For this review, use the dimensioned drawing (mm, ordinates from the lowest corner) and the shaded views. A direction names the side the tool comes from. Coordinates: 2 decimals unless noted, no trailing zeros. Loops run counter-clockwise (first coordinate to the right, second up) from the corner with the lowest first, then second, coordinate; pieces in that order, holes last. Notation, with made-up numbers: M 64,43 L 83,43 A31 ccw 83,71 Z; hole C 43.25,32.5 d5. An arc over 180 degrees is marked long. One line per item, written item: value.
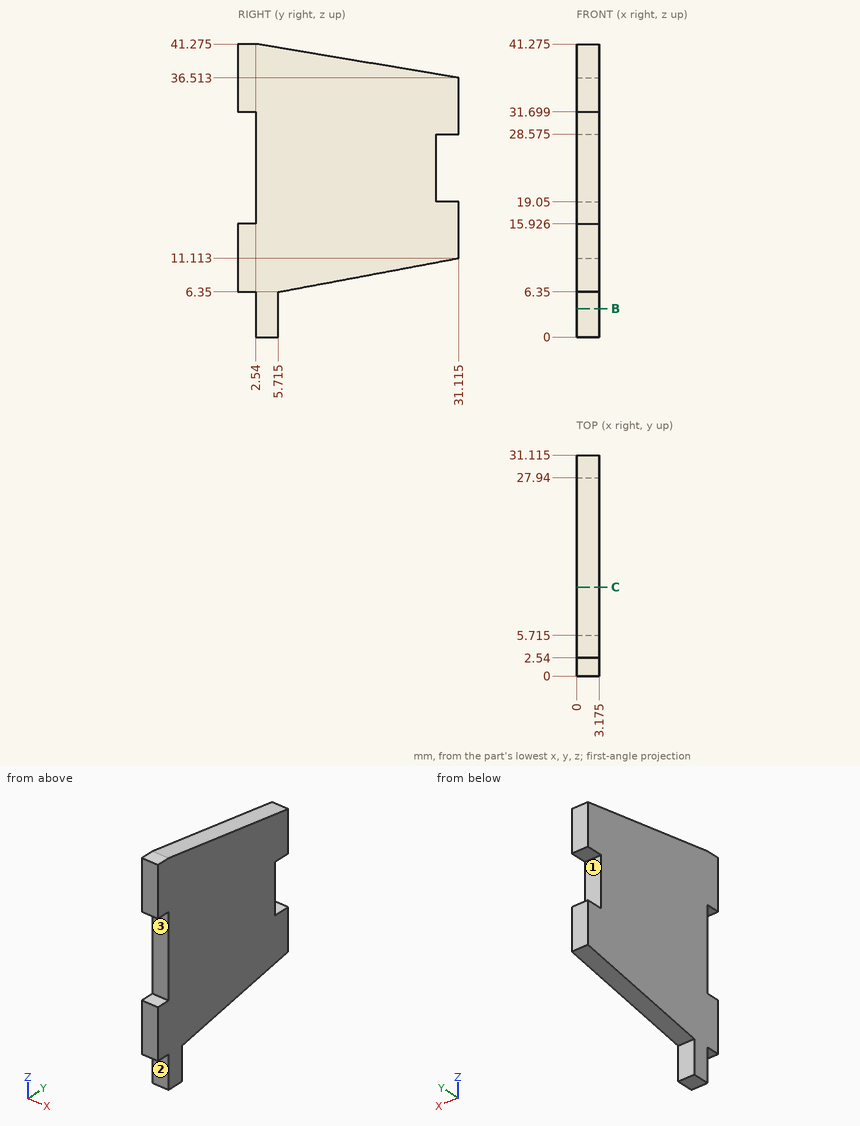
(1) We need section B-B on z = 4. State the section outline as (x, y) points (1 decimal).
Reply:
outline: M 0,2.5 L 3.2,2.5 L 3.2,5.7 L 0,5.7 Z
(2) We need section C-C on y = 12.5. State the section outline as (x, z) points (1 decimal).
Reply:
outline: M 0,7.6 L 3.2,7.6 L 3.2,39.6 L 0,39.6 Z
(3) To check wall thickness, follow line 1 along Y through (x, z) = (2.3, 29) (1 decimal); line 2 along Y through (x, z) = (0.85, 24); line 3 along Z through (x, y) = (1.35, 14) (1 decimal). State the ranges of each line that lie inside material, in increasing order. Write a range as [from, to].
Reply:
line 1: y = [2.5, 31.1]
line 2: y = [2.54, 27.94]
line 3: z = [7.9, 39.4]
(4) Tool access review of the marked faces 1, 2 and 3: name each direction out of +Z, -Z, +X, -X, +Y, -Y from which nothing blocks a thin tool from reaching the whole face with its end or side.
Reply:
face 1: +X, -X, +Y
face 2: -Z, +X, -X, -Y
face 3: +X, -X, -Y
(5) Insertion check: pin 1 (1 mm diameter, centred on x = 2, z = 4.5, fed in from -Y); pin 2 (1.6 mm diameter, centred on x = 1.5, y = 30.5, fed in from -Z); pin 3 (0.8 mm diameter, centred on x = 1, y = 1, fed in from -Z). Each pin has a flat end and moves straight along its axis. Give the tip position at first contact, or say it passes through.
Reply:
pin 1: stops at y = 2.54
pin 2: stops at z = 10.85
pin 3: stops at z = 6.35
